from build123d import *

# Parameters (mm, degrees)
ESQUISSE1_W             = 27
ESQUISSE1_H             = 71
BOSS_EXTRU_1_DEPTH      = 18
ESQUISSE2_R             = 1.65
ENL_V_MAT_EXTRU_1_DEPTH = 200.914193796
ESQUISSE5_R             = 2
BOSS_EXTRU_2_DEPTH      = 2.5
ESQUISSE6_R             = 2.5
ENL_V_MAT_EXTRU_2_DEPTH = 4
ESQUISSE7_R             = 1
ENL_V_MAT_EXTRU_3_DEPTH = 3
ESQUISSE7_3_R           = 1
ENL_V_MAT_EXTRU_4_DEPTH = 138.156023146
ESQUISSE8_R             = 2.5
ENL_V_MAT_EXTRU_5_DEPTH = 4


with BuildPart() as part:
    # Esquisse1 → Boss.-Extru.1 (new body)
    with BuildSketch(Plane(origin=(0, 0, 0), x_dir=(0, 0, -1), z_dir=(1, 0, 0))):
        with Locations((134.428733504, 97.762052682)):
            Rectangle(ESQUISSE1_W, ESQUISSE1_H)
    extrude(amount=BOSS_EXTRU_1_DEPTH)

    # Esquisse2 → Enl_v. mat.-Extru.1 (cut, through all)
    with BuildSketch(Plane.ZY):
        with Locations((-124.928733504, 97.262052682)):
            Circle(ESQUISSE2_R)
        with Locations((-124.928733504, 83.262052682)):
            Circle(ESQUISSE2_R)
    extrude(amount=-ENL_V_MAT_EXTRU_1_DEPTH, mode=Mode.SUBTRACT)

    # Esquisse5 → Boss.-Extru.2 (add)
    with BuildSketch(Plane(origin=(0, 0, -147.928733504), x_dir=(-1, 0, 0), z_dir=(0, 0, -1))):
        with Locations(Location((-9, 123.695505567, 0), (0, 0, 270))):
            Circle(ESQUISSE5_R)
    extrude(amount=BOSS_EXTRU_2_DEPTH)

    # Esquisse6 → Enl_v. mat.-Extru.2 (cut)
    with BuildSketch(Plane(origin=(0, 0, -147.928733504), x_dir=(-1, 0, 0), z_dir=(0, 0, -1))):
        with Locations((-10.5, 82.262052682)):
            Circle(ESQUISSE6_R)
        with Locations((-7.5, 98.262052682)):
            Circle(ESQUISSE6_R)
    extrude(amount=-ENL_V_MAT_EXTRU_2_DEPTH, mode=Mode.SUBTRACT)

    # Esquisse7 → Enl_v. mat.-Extru.3 (cut)
    # profile 1 of 4: a face of its own
    with BuildSketch(Plane(origin=(0, 0, -147.928733504), x_dir=(-1, 0, 0), z_dir=(0, 0, -1))):
        with BuildLine():
            Line((0, 108.562052682), (-2.5, 108.562052682))
            ThreePointArc((-2.5, 108.562052682), (-5.79996536, 105.277172969), (-2.530240256, 101.962191242))
            Line((-2.530240256, 101.962191242), (0, 101.962191242))
            Line((0, 101.962191242), (0, 108.562052682))
        make_face()
        with Locations((-2.5, 105.262052682)):
            Circle(ESQUISSE7_R, mode=Mode.SUBTRACT)
    # profile 2 of 4: a face of its own
    with BuildSketch(Plane(origin=(0, 0, -147.928733504), x_dir=(-1, 0, 0), z_dir=(0, 0, -1))):
        with Locations((-2.5, 105.262052682)):
            Circle(ESQUISSE7_R)
    # profile 3 of 4: a face of its own
    with BuildSketch(Plane(origin=(0, 0, -147.928733504), x_dir=(-1, 0, 0), z_dir=(0, 0, -1))):
        with BuildLine():
            ThreePointArc((-15.451765432, 71.962405212), (-12.200088134, 75.286170611), (-15.5, 78.562052682))
            Line((-15.5, 78.562052682), (-18, 78.562052682))
            Line((-18, 78.562052682), (-18, 71.962405212))
            Line((-18, 71.962405212), (-15.451765432, 71.962405212))
        make_face()
        with Locations((-15.5, 75.262052682)):
            Circle(ESQUISSE7_R, mode=Mode.SUBTRACT)
    # profile 4 of 4: a face of its own
    with BuildSketch(Plane(origin=(0, 0, -147.928733504), x_dir=(-1, 0, 0), z_dir=(0, 0, -1))):
        with Locations((-15.5, 75.262052682)):
            Circle(ESQUISSE7_R)
    extrude(amount=-ENL_V_MAT_EXTRU_3_DEPTH, mode=Mode.SUBTRACT)

    # Esquisse7_3 → Enl_v. mat.-Extru.4 (cut, through all)
    with BuildSketch(Plane(origin=(0, 0, -147.928733504), x_dir=(-1, 0, 0), z_dir=(0, 0, -1))):
        with Locations((-2.5, 105.262052682)):
            Circle(ESQUISSE7_3_R)
        with Locations((-15.5, 75.262052682)):
            Circle(ESQUISSE7_3_R)
    extrude(amount=-ENL_V_MAT_EXTRU_4_DEPTH, mode=Mode.SUBTRACT)

    # Esquisse8 → Enl_v. mat.-Extru.5 (cut)
    with BuildSketch(Plane.XY.offset(-120.928733504)):
        with Locations((8, 76.262052682)):
            Circle(ESQUISSE8_R)
        with Locations((9, 90.262052682)):
            Circle(ESQUISSE8_R)
        with Locations((10, 104.262052682)):
            Circle(ESQUISSE8_R)
    extrude(amount=-ENL_V_MAT_EXTRU_5_DEPTH, mode=Mode.SUBTRACT)


solid = part.part
Part model, mm, in its own coordinate system. A direction names the side the tool comes from. Coordinates: 2 decimals unless noted, no trailing zeros. Order: outer loops, then holes, each group sorted by start corner. A loop starts at its lowest first (then second) coordinate and runs counter-clockwise, first axis right, second up.
(1) Slice it at D-D, the plane y = 107.5. Write the cut outline in (x, z).
Check sheet entries:
outline: (0, -144.93) - (4.93, -144.93) - (4.93, -147.93) - (18, -147.93) - (18, -120.93) - (0, -120.93) - close
(2) Tool access for faces 1 (the face through (1, 101.962, -146)), 2 (the face through (9.46, 101.82, -122.9)), 3 (the face through (8, 98, -143.929)): list every direction of +Z, -Z, +X, -X, +Y, -Y with a clear straight run to the whole face (end or side of a thin tool).
Check sheet entries:
face 1: -Z, -X
face 2: +Z
face 3: -Z
(3) Slice it at B-B, the plane y = 119. Write the cut outline in (x, z), and give its area (3 significant figures).
Check sheet entries:
outline: (0, -147.93) - (18, -147.93) - (18, -120.93) - (0, -120.93) - close
area: 486 mm2
(4) Pull direction X, two halves, no side cores. Call faces 4 (the face through (7.65, 125.17, -149.16)), 5 (the face through (9, 133.262, -134)), 6 (the face through (8.46, 87.82, -122.9)): pulls with the +X half, pulls with the -X half, needs draft (parallel to the pull), parting line crosses it, or undercut.
Check sheet entries:
face 4: parting line crosses it
face 5: needs draft
face 6: undercut
(5) Slice it at A-A, the plane x = 9. State how many separate pieces and enclosed holes the cut face has, and give its area (3 significant figures).
Check sheet entries:
separate pieces: 1
enclosed holes: 2
area: 1,820 mm2
(6) Probe L1, parallel to Y at x = 15.5, z = -137.75; L2, parallel to Y at x = 2.5, z = -127.5; L3, parallel to Z at x = 6.75, y = 111.5. List the from-to ranges inside material, lowest first.
Check sheet entries:
L1: y = 62.26 to 74.26, 76.26 to 133.26
L2: y = 62.26 to 104.26, 106.26 to 133.26
L3: z = -147.93 to -120.93
(7) Slice it at C-C, the plane y = 88.5. Write the cut outline in (x, z).
Check sheet entries:
outline: (0, -147.93) - (18, -147.93) - (18, -120.93) - (10.77, -120.93) - (10.77, -124.93) - (7.23, -124.93) - (7.23, -120.93) - (0, -120.93) - close
(8) Pin check, flat tips, straight feed: pin 1 Ø3 at (x, y) = (15.5, 74) entering from -Z; pin 2 Ø12 at (y, z) = (97, -126.5) entering from -X; pin 3 Ø4 at (x, y) = (7.5, 98.26) entering from -Z; pin 4 Ø4 at (x, y) = (9, 90.26) entering from +Z. Stop position of each tip, or through.
Check sheet entries:
pin 1: stops at z = -144.93
pin 2: stops at x = 0
pin 3: stops at z = -143.93
pin 4: stops at z = -124.93
